Autodesk Inventor part; units mm, degrees
ref_plane "YZ Plane" through (0, 0, 0) normal (1, 0, 0) x (0, 1, 0)
ref_plane "XZ Plane" through (0, 0, 0) normal (0, 1, 0) x (-1, 0, 0)
ref_plane "XY Plane" through (0, 0, 0) normal (0, 0, 1) x (1, 0, 0)
sketch "Sketch1" plane through (0, 0, 0) normal (0, 0, 1) x (1, 0, 0)
  circle A0 centre (0, 0) radius 25
  circle A1 centre (0, 18.7369) radius 5
  circle A2 centre (-18.7369, 0) radius 5
  circle A3 centre (0, -18.7369) radius 5
  circle A4 centre (18.7369, 0) radius 5
  dimension "d0" = 50
  dimension "d1" = 10
  dimension "d4" = 360
extrude "Extrusion1" add sketch "Sketch1" along normal blind 10
Could you check a few things on this model? Use its own coordinates, in mm. Coordinates: 2 decimals unless noted, no trailing zeros. Write each loop counter-clockwise with the first axis right and the second up, starting at its lowest first coordinate (ties: lowest second). Pieces come first, ordered by that corner, then holes. Notation, with made-up numbers: (21, 9.25) - (51, 9.25) arc R29 ccw to (51, 48.25) - close; hole circle Ø4 at (68.5, -10). An arc over 180 degrees is marked (long way). Put each result on its own line as item: value. Start each with the question number.
Q1. I'm going to push flat-ended pins straight in: P1, Ø5, axis at y = -5.5, z = 3.5, coming from the -X side; P2, Ø1.5, axis at y = 17, z = 5, coming from the -X side; P3, Ø4, axis at y = -16, z = 5.5, coming from the +X side. Where does each tip first touch, or does it pass through?
Q2. I want a section at A-A on x = 0. Write out the boundary of the cut face in (y, z), plus the area to 3 significant figures.
Q3. I want a section at C-C on x = 20. Write out the boundary of the cut face in (y, z).
Q4. Thinking about a two-plate mould opening in X: for faces 1 (the cylindrical face through (23.846, -7.509, 4.93)), 2 (the cylindrical face through (-0.65, 13.78, 4.93)), 3 (the flat face through (0, 0, 10)), which applies, pulls with the +X half, pulls with the -X half, needs draft (parallel to the pull), parting line crosses it, or undercut?
Q5. Please list where these lines run through material, in increasing order: L1, parallel to Y at x = 0, z = 5; L2, parallel to Y at x = -4, z = 3; L3, parallel to X at y = -20, z = 5.5.
Q6. I want a section at D-D on y = -22. Write out the boundary of the cut face in (x, z), plus the area to 3 significant figures.
Checks:
1. P1: x = -24.82
1. P2: x = -19
1. P3: x = 20.71
2. outline: (-25, 0) - (-23.74, 0) - (-23.74, 10) - (-25, 10) - close; (-13.74, 0) - (13.74, 0) - (13.74, 10) - (-13.74, 10) - close; (23.74, 0) - (25, 0) - (25, 10) - (23.74, 10) - close
2. area: 300 mm²
3. outline: (-15, 0) - (-4.84, 0) - (-4.84, 10) - (-15, 10) - close; (4.84, 0) - (15, 0) - (15, 10) - (4.84, 10) - close
4. face 1: parting line crosses it
4. face 2: undercut
4. face 3: needs draft
5. L1: -25 to -23.74, -13.74 to 13.74, 23.74 to 25
5. L2: -24.68 to -21.74, -15.74 to 15.74, 21.74 to 24.68
5. L3: -15 to -4.84, 4.84 to 15
6. outline: (-11.87, 0) - (-3.79, 0) - (-3.79, 10) - (-11.87, 10) - close; (3.79, 0) - (11.87, 0) - (11.87, 10) - (3.79, 10) - close
6. area: 162 mm²
